from build123d import *

# Parameters (mm, degrees)
CLIP_BODY_DEPTH                            = 15
PRISM_START                                = -0.6
PRISM_CANTILEVER_EXTRUDE_DEPTH             = 3
PRISM_CANTILEVER_EXTRUDE_FILLET_R          = 0.2
PRISM_CANTILEVER_EXTRUDE_FILLET_OF_PRISM_R = 0.2
GLOBAL_FILLET_R                            = 0.5


with BuildPart() as part:
    # Sketch1 → Clip Body (new, symmetric)
    with BuildSketch(Plane(origin=(0, 0, 0), x_dir=(0, 0, -1), z_dir=(1, 0, 0))):
        with BuildLine():
            Line((0, 0), (0, 50))
            Line((0, 50), (6, 50))
            Line((6, 50), (6, 48))
            ThreePointArc((6, 48), (4.661306176, 25), (6, 2))
            Line((6, 2), (6, 0))
            Line((6, 0), (3, 0))
            Line((3, 0), (3, 2))
            Line((3, 2), (4.238207846, 2))
            ThreePointArc((4.238207846, 2), (2.911306176, 25), (4.238207846, 48))
            Line((4.238207846, 48), (2, 48))
            Line((2, 48), (2, 0))
            Line((2, 0), (0, 0))
        make_face()
    extrude(amount=CLIP_BODY_DEPTH, both=True)

    # Sketch9 → Prism Cantilever Extrude (add)
    with BuildSketch(Plane.ZY.offset(15).offset(PRISM_START)):
        Polygon((1.7, 48.8), (1.7, 49), (1.5, 49.2), (1.3, 49.2), (1.3, 49), (0, 49), (0, 48.8), align=None)
        Polygon((1.3, 1), (0, 1), (0, 1.2), (1.7, 1.2), (1.7, 1), (1.5, 0.8), (1.3, 0.8), align=None)
    prism_cantilever_extrude = extrude(amount=-PRISM_CANTILEVER_EXTRUDE_DEPTH)

    # Prism Cantilever Extrude Fillet
    prism_cantilever_extrude_fillet_edges = [part.edges().sort_by_distance(p)[0] for p in [
        (-12.9, 1, 0),
        (-12.9, 1.2, 0),
        (-12.9, 48.8, 0),
        (-12.9, 49, 0),
    ]]
    fillet(prism_cantilever_extrude_fillet_edges, radius=PRISM_CANTILEVER_EXTRUDE_FILLET_R)

    # Prism Cantilever Extrude Mirror: Prism Cantilever Extrude across plane
    add(prism_cantilever_extrude.mirror(Plane(origin=(0, 0, 0), x_dir=(0, 0, 1), z_dir=(1, 0, 0))))

    # Prism Cantilever Extrude Fillet of Prism
    prism_cantilever_extrude_fillet_of_prism_edges = [part.edges().sort_by_distance(p)[0] for p in [
        (12.9, 1, 0),
        (12.9, 1.2, 0),
        (12.9, 48.8, 0),
        (12.9, 49, 0),
    ]]
    fillet(prism_cantilever_extrude_fillet_of_prism_edges, radius=PRISM_CANTILEVER_EXTRUDE_FILLET_OF_PRISM_R)

    # Global Fillet
    global_fillet_edges = [part.edges().sort_by_distance(p)[0] for p in [
        (-15, 25, 0),
        (-15, 50, -3),
        (15, 48, -3.119103923),
        (-15, 49, -6),
        (-15, 25, -4.661306176),
        (-15, 1, -6),
        (-15, 0, -4.5),
        (-15, 1, -3),
        (-15, 2, -3.619103923),
        (-15, 25, -2.911306176),
        (-15, 48, -3.119103923),
        (-15, 24, -2),
        (-15, 0, -1),
        (15, 25, -2.911306176),
        (0, 0, 0),
        (0, 50, 0),
        (0, 50, -6),
        (15, 2, -3.619103923),
        (0, 48, -6),
        (0, 2, -6),
        (0, 0, -6),
        (0, 0, -3),
        (0, 2, -3),
        (0, 0, -2),
        (15, 1, -3),
        (15, 0, -4.5),
        (15, 1, -6),
        (15, 25, -4.661306176),
        (15, 49, -6),
        (15, 50, -3),
        (15, 25, 0),
        (15, 0, -1),
        (15, 24, -2),
    ]]
    fillet(global_fillet_edges, radius=GLOBAL_FILLET_R)


solid = part.part
The model under review builds one solid part; all positions refer to its coordinate system, in mm. A direction names the side the tool comes from. Give positions to 0.01 mm unless a question says otherwise; leave off trailing zeros. Loops run counter-clockwise (first coordinate to the right, second up) from the corner with the lowest first, then second, coordinate; pieces in that order, holes last. Notation, with made-up numbers: (51.5, 34.25) -> (97.5, 34.25) arc R31 cw to (97.5, 62.25) -> close; hole circle Ø10 at (-34, -36). An arc over 180 degrees is marked (long way). Write each question's results on one line, items separated by ' | '.
1) Tool access review of faces 5 (the face through (15, 25, -4)), 6 (the face through (-13, 1.2, 1)), 7 (the face through (13, 1, 1)), 8 (the face through (0, 48, -3)), 9 (the face through (13, 49, 1)): name each direction out of +Z, -Z, +X, -X, +Y, -Y from which nothing blocks a thin tool from reaching the whole face with its end or side.
Conclusion:
face 5: +Z, -Z, +X, +Y, -Y | face 6: +Z, +X, -X | face 7: +X, -X, -Y | face 8: +X, -X | face 9: +X, -X, +Y
2) Take a section at B-B, the plane x = -5. Give the boundary of the cut face in (y, z), plus the area to 3 significant figures.
Conclusion:
outline: (0, -5.5) arc R0.5 ccw to (0.5, -6) -> (1.97, -6) arc R0.5 ccw to (2.03, -6) arc R198.25 cw to (47.97, -6) arc R0.5 ccw to (48.03, -6) -> (49.5, -6) arc R0.5 ccw to (50, -5.5) -> (50, -0.5) arc R0.5 ccw to (49.5, 0) -> (0.5, 0) arc R0.5 ccw to (0, -0.5) -> (0, -1.5) arc R0.5 ccw to (0.5, -2) -> (48, -2) -> (48, -4.24) arc R200 ccw to (2, -4.24) -> (2, -3.5) arc R0.5 ccw to (1.5, -3) -> (0.5, -3) arc R0.5 ccw to (0, -3.5) -> close | area: 194 mm^2
3) Take a section at A-A, the plane z = 0.75. Give the boundary of the cut face in (x, y).
Conclusion:
outline: (-14.4, 1) -> (-11.4, 1) -> (-11.4, 1.2) -> (-14.4, 1.2) -> close; (-14.4, 48.8) -> (-11.4, 48.8) -> (-11.4, 49) -> (-14.4, 49) -> close; (11.4, 1) -> (14.4, 1) -> (14.4, 1.2) -> (11.4, 1.2) -> close; (11.4, 48.8) -> (14.4, 48.8) -> (14.4, 49) -> (11.4, 49) -> close
4) For line 1 along X through (y, z) = (22, -4.25); line 2 along Z through (x, y) = (-5.5, 40); line 3 along Z through (x, y) = (-1.5, 22), list the stretches that pass through material, from the lowest coordinate up. Write a range as from..to.
Conclusion:
line 1: x = -15..15 | line 2: z = -5.23..-3.47, -2..0 | line 3: z = -4.68..-2.93, -2..0
5) Draft analysis for pull direction Y (two halves, no side actions). For faces 1 (the face through (-13, 49, 1)), 2 (the face through (13, 1.2, 1)), 3 (the face through (0, 49, -6)), 4 (the face through (0.2, 25.32, -4.66)), state which applies: pulls with the +Y half, pulls with the -Y half, needs draft (parallel to the pull), parting line crosses it, or undercut.
Conclusion:
face 1: pulls with the +Y half | face 2: undercut | face 3: needs draft | face 4: undercut
6) Insertion check: pin 1 Ø0.5 at (y, z) = (49, 0.5) entering from +X; pin 2 Ø0.5 at (y, z) = (49, 1) entering from -X; pin 3 Ø14.5 at (x, y) = (-1, 21.5) entering from +Z. Each pin has a flat end and moves straight along its axis. Give the tip position at first contact, or say it passes through.
Conclusion:
pin 1: stops at x = 14.4 | pin 2: stops at x = -14.4 | pin 3: stops at z = 0
